Here's how the part is built. I have some questions about the finished solid (model axes, mm). Give positions to 0.01 mm unless a question says otherwise; leave off trailing zeros. Loops run counter-clockwise (first coordinate to the right, second up) from the corner with the lowest first, then second, coordinate; pieces in that order, holes last.
Q1. I need wall thicknesses on probe 1 along X at (y, z) = (-793, 158.5); probe 2 along Z at (x, y) = (250.5, -862.5). Which ranges of each line are inside material? Lowest first, please.
Q2. I'm going to push flat-ended pins straight in: P1, Ø1.5, axis at x = 258, y = -368, coming from the +Z side; P2, Ø12, axis at y = -1059, z = 155.5, coming from the -X side. Where does each tip first touch, or does it pass through?
Q3. Suppose I cut it at A-A (y = -1002). List the corners of the cut face in (x, z) for me, and give its area (4 significant figures).
Q4. Suppose I cut it at B-B (x = 266). List the corners of the cut face in (y, z) for me.
Q5. Suppose I cut it at C-C (z = 156.75). List the corners of the cut face in (x, y) for me.
Q6. Thinking about a two-plate mould opening in Y: for faces 1 (the face through (268, 75, 144)), 2 (the face through (262, -762, 143.5)), 3 (the face through (268, -1575, 144)), which applies, pulls with the +Y half, pulls with the -Y half, needs draft (parallel to the pull), parting line crosses it, or undercut?
```python
from build123d import *

# Parameters (mm, degrees)
BOSS_EXTRUDE1_DEPTH = 825


with BuildPart() as part:
    # Sketch2 → Boss-Extrude1 (new, symmetric)
    with BuildSketch(Plane.XZ.offset(750)):
        Polygon((275, 169.5), (273.5, 169.5), (273.5, 145), (249, 145), (249, 143.5), (275, 143.5), align=None)
    extrude(amount=BOSS_EXTRUDE1_DEPTH, both=True)


solid = part.part
```
Solutions:
1. probe 1: x = 273.5 to 275
1. probe 2: z = 143.5 to 145
2. P1: stops at z = 145
2. P2: stops at x = 273.5
3. outline: (249, 143.5) - (275, 143.5) - (275, 169.5) - (273.5, 169.5) - (273.5, 145) - (249, 145) - close
3. area: 75.75 mm2
4. outline: (-1575, 143.5) - (75, 143.5) - (75, 145) - (-1575, 145) - close
5. outline: (273.5, -1575) - (275, -1575) - (275, 75) - (273.5, 75) - close
6. face 1: pulls with the +Y half
6. face 2: needs draft
6. face 3: pulls with the -Y half
